Geometry check sheet. Reference: the model listing, model coordinates, mm. A direction names the side the tool comes from. Round coordinates to 2 decimals unless told otherwise and drop trailing zeros. Loops run counter-clockwise (first coordinate to the right, second up) from the corner with the lowest first, then second, coordinate; pieces in that order, holes last. Notation, with made-up numbers: (61, 44.5) -> (102, 44.5) arc R23 cw to (102, 59.5) -> close; hole circle Ø4 at (4, -8.5). An arc over 180 degrees is marked (long way). Use a Markdown table: item, result. Add a question column.
Q1. Set-up check for faces 1 (the face through (0.176, -13.504, 16.985)), 2 (the face through (7.62, -3.16, 11.15)): record each of +Z, -Z, +X, -X, +Y, -Y from which the full face is reachable in a straight line by a thin tool's end or side.
Q2. Sectioned sample at A-A, the plane x = 0. Give the number of separate pieces and of enclosed holes in the cut face, then the cut area to 3 significant figures.
Q3. Sectioned sample at C-C, the plane z = 10.75. Enter the section's corners in (x, y), then the cut area to 3 significant figures.
Q4. Material ranges on L1, parallel to X at y = -1.5, z = 21; L2, parallel to X at y = -1, z = 16.5; L3, parallel to Z at x = -17, y = -13.5, recorded low to high.
Q5. Sectioned sample at D-D, the plane x = 6. Enter the section's corners in (y, z), then the cut area to 3 significant figures.
Q6. Gauge pin test, flat ends, axial feed: P1, Ø3.5, axis at x = -17.5, y = 0, coming from the +Z side; P2, Ø7, axis at x = 17.5, y = 0, coming from the -Z side; P3, Ø9, axis at x = 1.5, y = -18, coming from the -Z side; P4, Ø5, axis at y = -3, z = 18, coming from the +X side. Record the tip position at first contact, or that the pin passes through.
Q7. Release check for a two-part mould opening along X. For faces 3 (the face through (10.382, -19.961, 18.451)), 4 (the face through (3, -8, 0)), 5 (the face through (0.676, -19.646, 20.479)) record: released by +X, released by -X, zero draft, split by the parting line, or undercut.
```python
from build123d import *

# Parameters (mm, degrees)
SKETCH_1_R               = 12.5
EXTRUDE_1_DEPTH          = 15
SKETCH_2_R               = 22.5
EXTRUDE_2_DEPTH          = 7
M18X1_5_1_D              = 16.5
M18X1_5_1_DEPTH          = 43.5
M18X1_5_1_TIP            = 4.957100107
PATTERN_CIRCULAR_1_COUNT = 4


with BuildPart() as part:
    # 草图1 → 拉伸1 (new body)
    with BuildSketch(Plane.XY):
        Circle(SKETCH_1_R)
    extrude(amount=EXTRUDE_1_DEPTH)

    # 草图2 → 拉伸2 (add)
    with BuildSketch(Plane.XY.offset(15)):
        Circle(SKETCH_2_R)
    extrude(amount=EXTRUDE_2_DEPTH)

    # M18x1.5 螺纹孔1
    with Locations(Plane(origin=(0, 0, 0), x_dir=(-1, 0, 0), z_dir=(0, 0, -1))):
        with Locations((0, 0)):
            Hole(M18X1_5_1_D / 2, depth=M18X1_5_1_DEPTH)
            with Locations((0, 0, -(M18X1_5_1_DEPTH + M18X1_5_1_TIP / 2))):  # 118° drill point
                Cone(0, M18X1_5_1_D / 2, M18X1_5_1_TIP, mode=Mode.SUBTRACT)

    # 草图5 → M4 六角凹头螺钉的柱形沉头孔1 (revolve, cut)
    with BuildSketch(Plane(origin=(0, 17.5, 15), x_dir=(0, 1, 0), z_dir=(1, 0, 0))):
        Polygon((0, 0), (0, 7), (2.25, 7), (2.25, 4), (4, 4), (4, 0.025), (4.025, 0), align=None)
    hole_wizard_m4_1 = revolve(axis=Axis((0, 17.5, 8.65), (0, 0, 1)), mode=Mode.SUBTRACT)

    # 阵列(圆周)1: M4 六角凹头螺钉的柱形沉头孔1 ×4 about axis
    pattern_circular_1_axis = Axis((0, 0, 0), (0, 0, 1))
    for i in range(1, PATTERN_CIRCULAR_1_COUNT):
        add(hole_wizard_m4_1.rotate(pattern_circular_1_axis, i * 360 / PATTERN_CIRCULAR_1_COUNT), mode=Mode.SUBTRACT)


solid = part.part
```
Values:
| question | item | result |
|---|---|---|
| 1 | face 1 | -Z |
| 1 | face 2 | +Z, -Z |
| 2 | separate pieces | 4 |
| 2 | enclosed holes | 0 |
| 2 | area | 236 mm^2 |
| 3 | outline | circle Ø25 at (0, 0); hole circle Ø16.5 at (0, 0) |
| 3 | area | 277 mm^2 |
| 4 | L1 | -22.45 to -19.18, -15.82 to -8.11, 8.11 to 15.82, 19.18 to 22.45 |
| 4 | L2 | -22.48 to -21.37, -13.63 to -8.19, 8.19 to 13.63, 21.37 to 22.48 |
| 4 | L3 | 15 to 22 |
| 5 | outline | (-21.69, 15) -> (-10.97, 15) -> (-10.97, 0) -> (-5.66, 0) -> (-5.66, 22) -> (-21.69, 22) -> close; (5.66, 0) -> (10.97, 0) -> (10.97, 15) -> (21.69, 15) -> (21.69, 22) -> (5.66, 22) -> close |
| 5 | area | 383 mm^2 |
| 6 | P1 | through |
| 6 | P2 | z = 19 |
| 6 | P3 | z = 15 |
| 6 | P4 | x = 22.49 |
| 7 | face 3 | split by the parting line |
| 7 | face 4 | zero draft |
| 7 | face 5 | undercut |
